CAD build for the part. Positions are in the model's coordinates, mm. A direction names the side the tool comes from. Round coordinates to 2 decimals unless told otherwise and drop trailing zeros. Loops run counter-clockwise (first coordinate to the right, second up) from the corner with the lowest first, then second, coordinate; pieces in that order, holes last. Notation, with made-up numbers: M -20.5,23.5 L 30.5,23.5 A10 ccw 30.5,42.5 Z; hole C 17.5,-0.75 d5. An arc over 180 degrees is marked long. One line per item, written item: value. Start each with the question number.
Autodesk Inventor part; units mm, degrees
ref_plane "Work Plane1" through (66.6877, 0, 0) normal (0, 0, -1) x (1, 0, 0)
ref_plane "YZ Plane" through (0, 0, 0) normal (1, 0, 0) x (0, 1, 0)
ref_plane "XZ Plane" through (0, 0, 0) normal (0, 1, 0) x (-1, 0, 0)
sketch "Sketch1" plane through (0, 0, 0) normal (0, 0, 1) x (1, 0, 0)
  line L0 (12.7, 0) -> (12.7, 1.7526)
  line L1 (12.7, 1.7526) -> (2.4638, 1.7526)
  line L2 (0, 3.3401) -> (0, 1.2192)
  line L3 (0, 1.2192) -> (1.6764, 1.2192)
  line L4 (1.6764, 1.2192) -> (2.3803, 0)
  line L5 (2.3803, 0) -> (12.7, 0)
  line L6 (0, 3.3401) -> (0.6376, 3.3401)
  line L7 (0.6376, 3.3401) -> (2.4638, 1.7526)
  line L8 (-2.54, 0) -> (15.24, 0)
  line L9 (0, -0.668) -> (0, 4.0081)
  dimension "d0" = 12.7
  dimension "d1" = 1.6764
  dimension "d2" = 3.5052
  dimension "d3" = 2.4638
  dimension "d4" = 41
  dimension "d5" = 2.4384
  dimension "d6" = 60
  dimension "d7" = 6.6802
revolve "Body" add sketch "Sketch1" angle 360 about axis through (2.3803, 0, 0) along (1, 0, 0) contours L5 L4 L3 L2 L6 L7 L1 L0
sketch "Sketch2" plane through (0, 0, 0) normal (-1, 0, 0) x (0, 0, 1)
  circle A0 centre (0, 0) radius 3.3401
  circle A1 centre (0, 0) radius 1.2192
  line L0 (0.9421, 0.2524) -> (1.1777, 0.3156)
  line L1 (0.9421, -0.2524) -> (1.1777, -0.3156)
  arc A2 (0.9421, -0.2524) -> (0.9421, 0.2524) centre (0, 0) ccw
  arc A3 (1.1777, -0.3156) -> (1.1777, 0.3156) centre (0, 0) ccw
  line L2 (0, -4.6761) -> (0, 4.6761)
  line L3 (-4.6761, 0) -> (4.6761, 0)
  line L4 (0.9421, 0.2524) -> (0, 0) construction
  line L5 (0, 0) -> (0.9421, -0.2524) construction
  line L6 (0.2524, 0.9421) -> (0.3156, 1.1777)
  line L7 (0.6897, 0.6897) -> (0.8621, 0.8621)
  arc A4 (0.6897, 0.6897) -> (0.2524, 0.9421) centre (0, 0) ccw
  arc A5 (0.8621, 0.8621) -> (0.3156, 1.1777) centre (0, 0) ccw
  line L8 (-0.6897, 0.6897) -> (-0.8621, 0.8621)
  line L9 (-0.2524, 0.9421) -> (-0.3156, 1.1777)
  arc A6 (-0.2524, 0.9421) -> (-0.6897, 0.6897) centre (0, 0) ccw
  arc A7 (-0.3156, 1.1777) -> (-0.8621, 0.8621) centre (0, 0) ccw
  line L10 (-0.9421, -0.2524) -> (-1.1777, -0.3156)
  line L11 (-0.9421, 0.2524) -> (-1.1777, 0.3156)
  arc A8 (-0.9421, 0.2524) -> (-0.9421, -0.2524) centre (0, 0) ccw
  arc A9 (-1.1777, 0.3156) -> (-1.1777, -0.3156) centre (0, 0) ccw
  line L12 (-0.2524, -0.9421) -> (-0.3156, -1.1777)
  line L13 (-0.6897, -0.6897) -> (-0.8621, -0.8621)
  arc A10 (-0.6897, -0.6897) -> (-0.2524, -0.9421) centre (0, 0) ccw
  arc A11 (-0.8621, -0.8621) -> (-0.3156, -1.1777) centre (0, 0) ccw
  line L14 (0.6897, -0.6897) -> (0.8621, -0.8621)
  line L15 (0.2524, -0.9421) -> (0.3156, -1.1777)
  arc A12 (0.2524, -0.9421) -> (0.6897, -0.6897) centre (0, 0) ccw
  arc A13 (0.3156, -1.1777) -> (0.8621, -0.8621) centre (0, 0) ccw
  dimension "d8" = 1.9507
  dimension "d9" = 2.4384
  dimension "d10" = 15
  dimension "d11" = 15
  dimension "d22" = 360
extrude "Slot" add sketch "Sketch2" against normal up to next contours L3 A2 L0 A1 | A1 L1 A2 L3 | L3 A8 L10 A1 | A1 L11 A8 L3 | A1 L7 A4 L6 | L9 A6 L8 A1 | A1 L13 A10 L12 | L15 A12 L14 A1
thread "Thread"
chamfer "Chamfer1" distance 0.4724 distance2 0.9449 1 edges at (12.7, -1.7526, 0) measured on face at (12.7, 0.5842, 0.7748)
ref_plane "Work Plane1" through (66.6877, 0, 0) normal (0, 0, -1) x (1, 0, 0)
equation "\"d0\" = NLG"
equation "\"d1\" = INTI"
equation "\"d2\" = GD"
equation "\"d3\" = KOH"
equation "\"d4\" = 0.5 * SEWI"
equation "\"d5\" = SW"
equation "\"d7\" = KOD"
equation "\"d8\" = 0.8 * SW"
equation "\"d9\" = SW"
equation "\"d15\" = GEL"
equation "\"d17\" = -0.5 * SPD + 0.5 * GD"
equation "\"d18\" = GUL"
equation "\"NLG\" = 12.7"
equation "\"SW\" = 2.4384"
equation "\"INTI\" = 1.6764"
equation "\"GEL\" = 8.25195"
equation "\"KOH\" = 2.4638"
equation "\"KOD\" = 6.6802"
equation "\"GUL\" = 0.94488"
equation "\"SPD\" = 2.56032"
equation "\"GD\" = NND"
equation "\"SEWI\" = 82deg"
equation "\"TOA\" = 30deg"
equation "\"GD1\" = SPD"
equation "\"EPV\" = 4.4794"
equation "\"THREADDIA\" = 3.5052"
equation "\"BDM\" = NND"
equation "\"NND\" = 3.5052"
equation "\"GAL\" = 1.9845"
equation "\"E0\" = 1.155 * SW"
properties part number "ANSI B18.3 - 6-32 UNC x 0.5, SSFCHCSI" material "Steel, Mild"
(1) Which spindle directions (+Z, -Z, +X, -X, +Y, -Y) get a long thin tool onto all of the face, cutting with end or side? Do faces 4 (the cylindrical face through (7.04, 1.67, -0.53)), 5 (the flat face through (0, -1, -1)). Say none if no direction does.
(2) Slice it at A-A, the plane x = 10.75. List the corners of the cut face in (y, z).
(3) Probe L1, parallel to Z at x = 9.5, y = -1.5; L2, parallel to Z at x = 5.5, y = -1.25. List the from-to ranges inside material, lowest first.
(4) Mould opens along Y. For faces 1 (the flat face through (12.7, 0, 0)), 2 (the conical face through (2.34, -0.02, 0.07)), 3 (the cylindrical face through (0.323, 1.796, 2.816)) say: pulls with the +Y half, pulls with the -Y half, needs draft (parallel to the pull), parting line crosses it, or undercut.
(5) Flat gauge pins, fed straight in: P1, Ø4, axis at x = 3.5, z = 2, coming from the -Y side; P2, Ø2, axis at x = 10.5, y = 0.5, coming from the -Z side; P3, Ø3, axis at y = 2, z = 1, coming from the -X side; P4, Ø2, axis at x = 1.5, y = 2, coming from the -Z side. Where does each tip first touch, or does it go through?
Check result:
1. face 4: +X
1. face 5: +Z, -Z, -X, +Y, -Y
2. outline: C 0,0 d3.51
3. L1: z = -0.91 to 0.91
3. L2: z = -1.23 to 1.23
4. face 1: needs draft
4. face 2: undercut
4. face 3: parting line crosses it
5. P1: stops at y = -2.14
5. P2: stops at z = -1.75
5. P3: stops at x = 0
5. P4: stops at z = -2.99
